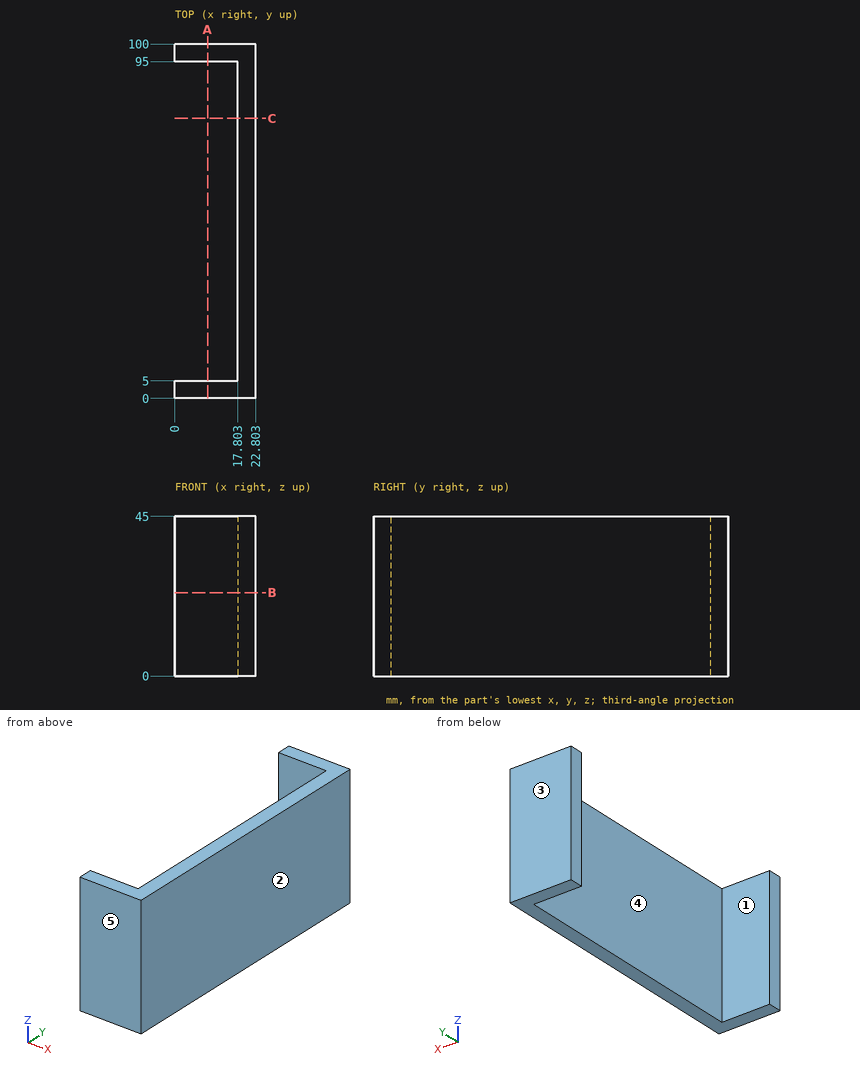
Answer from the drawing. Dimensions are ordinates in mm from the lowest x, y and z of the part. A direction names the side the tool comes from. Give positions to 0.01 mm unless a question says otherwise; leave off trailing zeros. Loops run counter-clockwise (first coordinate to the right, second up) from the corner with the lowest first, then second, coordinate; pieces in that order, holes last.
Item 1: Find the intervals of material crossed by line 1 along Y through (x, z) = (3, 41); line 2 along X through (y, z) = (21, 20.5), in increasing order.
Item 2: The mould has two halves that part along Y. Classify the marked faces 1, 2 and 3: released by +Y, released by -Y, zero draft, split by the parting line, or undercut.
Item 3: The part is cut by section C-C (y = 79). Write down the section's boundary in (x, z), and give its area (3 significant figures).
Item 4: The part is cut by section B-B (z = 23.5). Write down the section's boundary in (x, y), and give its area (3 significant figures).
Item 5: For the marked faces 4 and 5, determine the directions among +Z, -Z, +X, -X, +Y, -Y from which every point of the face is accessible in a straight line to the end or side of a thin tool.
Item 6: This flat-tipped pin is pushed along its axis until it touches: pin 1 Ø6 at (y, z) = (77, 35.5) entering from -X. Where does it stop, or does it pass through?
Item 7: The part is cut by section A-A (x = 9.25). Write down the section's boundary in (y, z).
Taken from the geometry:
1. line 1: y = 0 to 5, 95 to 100
1. line 2: x = 17.8 to 22.8
2. face 1: undercut
2. face 2: zero draft
2. face 3: released by +Y
3. outline: (17.8, 0) - (22.8, 0) - (22.8, 45) - (17.8, 45) - close
3. area: 225 mm2
4. outline: (0, 0) - (22.8, 0) - (22.8, 100) - (0, 100) - (0, 95) - (17.8, 95) - (17.8, 5) - (0, 5) - close
4. area: 678 mm2
5. face 4: +Z, -Z, -X
5. face 5: +Z, -Z, +X, -X, -Y
6. pin 1: stops at x = 17.8
7. outline: (0, 0) - (5, 0) - (5, 45) - (0, 45) - close; (95, 0) - (100, 0) - (100, 45) - (95, 45) - close
